from build123d import *

# Parameters (mm, degrees)
PAD_DEPTH    = 9
SKETCH001_W  = 26.1
SKETCH001_H  = 34.4
POCKET_DEPTH = 3
SKETCH002_R  = 22.22
PAD001_DEPTH = 3
SKETCH003_R  = 24.44
PAD002_DEPTH = 3
SKETCH004_R  = 26.6
PAD003_DEPTH = 3
SKETCH005_R  = 28
PAD004_DEPTH = 3


with BuildPart() as part:
    # Sketch → Pad (new body)
    with BuildSketch(Plane.XY):
        Polygon((44, 0), (22, 38.105118), (-22, 38.105118), (-44, 0), (-22, -38.105118), (22, -38.105118), align=None)
    extrude(amount=PAD_DEPTH)

    # Sketch001 (on Face8 of Pad) → Pocket (cut)
    with BuildSketch(Plane.XY.offset(9)):
        with Locations((0, -13.905118)):
            Rectangle(SKETCH001_W, SKETCH001_H)
    extrude(amount=-POCKET_DEPTH, mode=Mode.SUBTRACT)

    # Sketch002 (on Face5 of Pocket) → Pad001 (join)
    with BuildSketch(Plane.XY.offset(9)):
        Polygon((22, 38.105118), (-22, 38.105118), (-44, 0), (-22, -38.105118), (22, -38.105118), (44, 0), align=None)
        Circle(SKETCH002_R, mode=Mode.SUBTRACT)
    extrude(amount=PAD001_DEPTH)

    # Sketch003 (on Face14 of Pad001) → Pad002 (join)
    with BuildSketch(Plane.XY.offset(12)):
        Polygon((40, 0), (20, 34.641016), (-20, 34.641016), (-40, 0), (-20, -34.641016), (20, -34.641016), align=None)
        Circle(SKETCH003_R, mode=Mode.SUBTRACT)
    extrude(amount=PAD002_DEPTH)

    # Sketch004 (on Face21 of Pad002) → Pad003 (join)
    with BuildSketch(Plane.XY.offset(15)):
        Polygon((41, 0), (20.5, 35.507042), (-20.5, 35.507042), (-41, 0), (-20.5, -35.507042), (20.5, -35.507042), align=None)
        Circle(SKETCH004_R, mode=Mode.SUBTRACT)
    extrude(amount=PAD003_DEPTH)

    # Sketch005 (on Face28 of Pad003) → Pad004 (join)
    with BuildSketch(Plane.XY.offset(18)):
        Polygon((19, 32.908965), (-19, 32.908965), (-38, 0), (-19, -32.908965), (19, -32.908965), (38, 0), align=None)
        Circle(SKETCH005_R, mode=Mode.SUBTRACT)
    extrude(amount=PAD004_DEPTH)


solid = part.part
Can you work these out from the model? Positions are in its coordinate system, mm. A direction names the side the tool comes from. Give positions to 0.01 mm unless a question says otherwise; leave off trailing zeros. Write each loop counter-clockwise with the first axis right and the second up, starting at its lowest first coordinate (ties: lowest second). Pieces come first, ordered by that corner, then holes. Notation, with made-up numbers: M 61.25,4 L 111.25,4 A14 cw 111.25,10 Z; hole C -29,-14.5 d2. An arc over 180 degrees is marked long. Answer in a Markdown table with one row per item. Add a question column.
Item 1: On a 3-axis mill with a long thin cutter (end or side, diameter ignored), from which of +Z, -Z, +X, -X, +Y, -Y can I reach the whole of each face in a straight line? I mean faces 4 (the flat face through (28.633, 16.224, 19.479)), 5 (the flat face through (0, 7, 9)), 6 (the flat face through (0, -35.507, 16)). Say none if no direction works.
Item 2: Please list where these lines run through material, in increasing order: L1, parallel to Y at x = 0, z = 19.95; L2, parallel to Y at x = -2, z = 6.5; L3, parallel to Z at x = -23, y = -34.5.
Item 3: Imagine slicing it at A-A, the plane z = 16.75. Write out the boundary of the cut face in (x, y).
Item 4: For pin 1 Ø0.9 at (y, z) = (-12, 7.5) entering from +X; pin 2 Ø4 at (y, z) = (29.5, 15) entering from +X; pin 3 Ø4 at (y, z) = (-0.5, 2.5) entering from +X, each with a flat end and sliding along its axis, tell me the tip position at first contact or that it passes through.
Item 5: Imagine slicing it at B-B, the plane z = 4.75. Write out the boundary of the cut face in (x, y).
Item 6: We'd pull the mould along X, two halves only. Please class faces 1 (the flat face through (0, 35.507, 16)), 2 (the cylindrical face through (-17.633, -13.521, 10.479)), 3 (the flat face through (32.846, -19.319, 5.916)): released by +X, released by -X, zero draft, split by the parting line, or undercut.
Evaluation:
| question | item | result |
|---|---|---|
| 1 | face 4 | +Z, +X, +Y |
| 1 | face 5 | +Z |
| 1 | face 6 | +Z, +X, -X, -Y |
| 2 | L1 | y = -32.91 to -28, 28 to 32.91 |
| 2 | L2 | y = -38.11 to -31.11, 3.29 to 38.11 |
| 2 | L3 | z = 0 to 12 |
| 3 | outline | M -41,0 L -20.5,-35.51 L 20.5,-35.51 L 41,0 L 20.5,35.51 L -20.5,35.51 Z; hole C 0,0 d53.2 |
| 4 | pin 1 | stops at x = 37.33 |
| 4 | pin 2 | stops at x = 25.12 |
| 4 | pin 3 | stops at x = 44 |
| 5 | outline | M -44,0 L -22,-38.11 L 22,-38.11 L 44,0 L 22,38.11 L -22,38.11 Z |
| 6 | face 1 | zero draft |
| 6 | face 2 | undercut |
| 6 | face 3 | released by +X |
